from build123d import *

# Parameters (mm, degrees)
F0_W      = 50.8
F0_H      = 29.21
F1_DEPTH  = 123.698
F3_DEPTH  = 123.698
F4_W      = 98.298
F4_H      = 10.795
F5_DEPTH  = 50.8
F6_W      = 98.298
F6_H      = 28.448
F7_DEPTH  = 98.298
F10_DEPTH = 9.398
F11_DEPTH = 9.398
F12_W     = 9.398
F12_H     = 9.398
F13_DEPTH = 98.298
F14_W     = 57.15
F14_H     = 9.398
F15_DEPTH = 98.298
F16_R     = 9.525
F17_DEPTH = 28.448


with BuildPart() as f1:
    # F0 (on Right) → F1 (new body)
    with BuildSketch(Plane.YZ):
        with Locations((15.4936162289, 40.8715208429)):
            Rectangle(F0_W, F0_H)
    extrude(amount=F1_DEPTH)

    # F2 (on face) → F3 (cut)
    with BuildSketch(Plane.YZ.offset(123.698)):
        Polygon((23.3676162289, 46.0785208429), (23.3676162289, 55.4765208429), (7.6196162289, 55.4765208429), (7.6196162289, 46.0785208429), (0, 46.0785208429), (0, 38.2045208429), (31.3686162289, 38.2045208429), (31.3686162289, 46.0785208429), align=None)
    extrude(amount=-F3_DEPTH, mode=Mode.SUBTRACT)

    # F4 (on face) → F5 (join)
    with BuildSketch(Plane.XZ.offset(9.9063837711)):
        with Locations((49.149, 20.8690208429)):
            Rectangle(F4_W, F4_H)
    extrude(amount=-F5_DEPTH)

    # F6 (on face) → F7 (join)
    with BuildSketch(Plane(origin=(0, 0, 0), x_dir=(0, -1, 0), z_dir=(-1, 0, 0))):
        with Locations((8.2553837711, 1.2475208429)):
            Rectangle(F6_W, F6_H)
    extrude(amount=-F7_DEPTH)

    # F9 (on face) → F10 (join)
    with BuildSketch(Plane.YZ.offset(98.298)):
        Polygon((-35.3063837711, 15.4715208429), (-9.9063837711, 15.4715208429), (-9.9063837711, 26.2665208429), (-9.9063837711, 40.8715208429), align=None)
    extrude(amount=-F10_DEPTH)

    # F8 (on face) → F11 (join)
    with BuildSketch(Plane(origin=(0, 0, 0), x_dir=(0, -1, 0), z_dir=(-1, 0, 0))):
        Polygon((9.9063837711, 40.8715208429), (9.9063837711, 15.4715208429), (35.3063837711, 15.4715208429), align=None)
    extrude(amount=-F11_DEPTH)

    # F12 (on face) → F13 (cut)
    with BuildSketch(Plane.YZ.offset(98.298)):
        with Locations((-52.7053837711, -8.2774791571)):
            Rectangle(F12_W, F12_H)
    extrude(amount=-F13_DEPTH, mode=Mode.SUBTRACT)

    # F14 (on face) → F15 (cut)
    with BuildSketch(Plane.YZ.offset(98.298)):
        with Locations((12.3186162289, -8.2774791571)):
            Rectangle(F14_W, F14_H)
    extrude(amount=-F15_DEPTH, mode=Mode.SUBTRACT)

    # F16 (on face) → F17 (cut)
    with BuildSketch(Plane.XY.offset(15.4715208429)):
        with Locations((49.022, -32.0043837711)):
            Circle(F16_R)
    extrude(amount=-F17_DEPTH, mode=Mode.SUBTRACT)


solid = f1.part
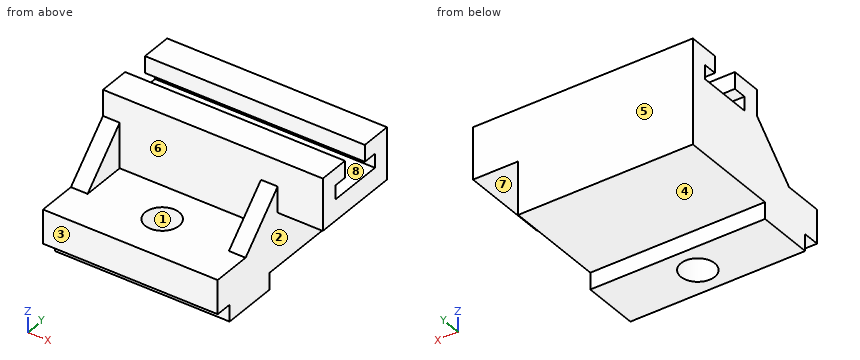
Design review of the part built by this model. Coordinates are the model's own, in mm. Face numbers are marked on the shaded views. A direction names the side the tool comes from. Round coordinates to 2 decimals unless told otherwise and drop trailing zeros. Write each loop counter-clockwise with the first axis right and the second up, starting at its lowest first coordinate (ties: lowest second). Pieces come first, ordered by that corner, then holes. Notation, with made-up numbers: M 59.5,-32.75 L 94.5,-32.75 A15 ccw 94.5,-22.75 Z; hole C -4.5,54.5 d10. An arc over 180 degrees is marked long. One line per item, written item: value. Start each with the question number.
1. Draft analysis for pull direction Y (two halves, no side actions). For the marked faces 1, 2 and 3, state which applies: pulls with the +Y half, pulls with the -Y half, needs draft (parallel to the pull), parting line crosses it, or undercut.
2. To check wall thickness, follow probe 1 along Y at (x, z) = (92.5, 44); probe 2 along Z at (x, y) = (28.5, 4); probe 3 along Y at (x, z) = (17.5, 47.5). State the ranges of each line that lie inside material, in increasing order. Write a range as from..to.
3. Take a section at B-B on x = 33.5. State the section outline as (y, z) points, then the cut area to 3 significant figures.
4. Take a section at C-C on z = 3. State the section outline as (x, y) points (3 decimals).
5. Take a section at A-A on y = 28.5. State the section outline as (x, z) points, then the cut area to 3 significant figures.
6. Take a section at D-D on x = 55. State the section outline as (y, z) points.
7. Clearance check with flat-ended pins moving along their axes: P1, Ø25, axis at x = 40, y = 15, coming from the +Z side; P2, Ø5, axis at x = 107.5, y = 0, coming from the -Z side; P3, Ø23.5, axis at x = 34, y = -31, coming from the +Z side; P4, Ø2, axis at x = 81.5, z = 28.5, coming from the -Y side. State where each tip first meets the part, or that it passes through.
8. For the marked faces 4, 5, 6, 7 and 8, list the 3-axis set-ups (+Z, -Z, +X, -X, +Y, -Y) from which the entire face can be reached by the end or side of a thin tool; tool diameter is ignored.
Computed:
1. face 1: undercut
1. face 2: needs draft
1. face 3: pulls with the -Y half
2. probe 1: y = -9.91..0, 31.37..40.89
2. probe 2: z = -3.58..38.2, 46.08..55.48
2. probe 3: y = -9.91..7.62, 23.37..40.89
3. outline: M -57.4,-3.58 L -48.01,-3.58 L -48.01,-12.98 L -16.26,-12.98 L -16.26,-3.58 L 40.89,-3.58 L 40.89,55.48 L 23.37,55.48 L 23.37,46.08 L 31.37,46.08 L 31.37,38.2 L 0,38.2 L 0,46.08 L 7.62,46.08 L 7.62,55.48 L -9.91,55.48 L -9.91,15.47 L -57.4,15.47 Z
3. area: 3,810 mm²
4. outline: M 0,-57.404 L 98.298,-57.404 L 98.298,40.894 L 0,40.894 Z; hole C 49.022,-32.004 d19.05
5. outline: M 0,-3.58 L 98.3,-3.58 L 98.3,26.27 L 123.7,26.27 L 123.7,38.2 L 0,38.2 Z; M 0,46.08 L 123.7,46.08 L 123.7,55.48 L 0,55.48 Z
5. area: 5,570 mm²
6. outline: M -57.4,-3.58 L -48.01,-3.58 L -48.01,-12.98 L -39.42,-12.98 L -39.42,15.47 L -57.4,15.47 Z; M -24.59,-12.98 L -16.26,-12.98 L -16.26,-3.58 L 40.89,-3.58 L 40.89,55.48 L 23.37,55.48 L 23.37,46.08 L 31.37,46.08 L 31.37,38.2 L 0,38.2 L 0,46.08 L 7.62,46.08 L 7.62,55.48 L -9.91,55.48 L -9.91,15.47 L -24.59,15.47 Z
7. P1: stops at z = 55.48
7. P2: stops at z = 26.27
7. P3: stops at z = 15.47
7. P4: stops at y = -9.91
8. face 4: -Z, +X, -X, +Y
8. face 5: +Z, -Z, +X, -X, +Y
8. face 6: +Z, -Y
8. face 7: -Z, +X, +Y, -Y
8. face 8: +X, -X
